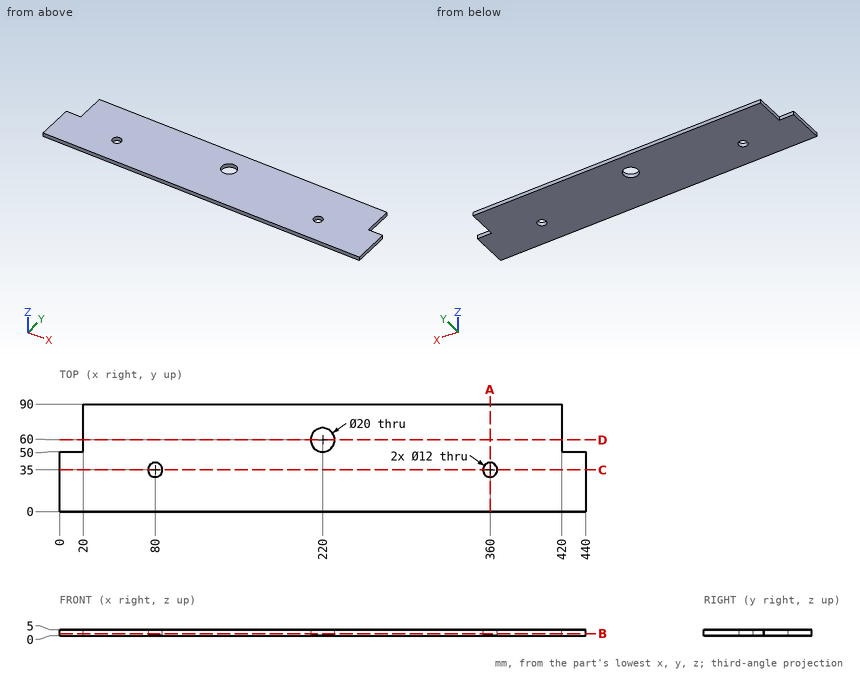
The figure shows three views and two pictorial views of one solid part (mm, origin at its lowest corner). Answer the questions. Give positions to 0.01 mm unless a question says otherwise; leave off trailing zeros. Write each loop counter-clockwise with the first axis right and the second up, starting at its lowest first coordinate (ties: lowest second). Pieces come first, ordered by that corner, then holes. Notation, with made-up numbers: (2.5, 59) -> (16.5, 59) arc R20 cw to (16.5, 75) -> close; hole circle Ø7 at (49, 7). An arc over 180 degrees is marked (long way). Answer as a JSON object with one key per item and string values.
1) Section A-A on x = 360 is taken. Write down the section's boundary in (y, z), then the cut area to 3 significant figures.
Findings below:
{"outline": "(0, 0) -> (29, 0) -> (29, 5) -> (0, 5) -> close; (41, 0) -> (90, 0) -> (90, 5) -> (41, 5) -> close", "area": "390 mm^2"}
2) Flat-ended cylindrical pins translate along their axes: pin 1 Ø16 at (x, y) = (220, 60) entering from -Z; pin 2 Ø2.5 at (x, z) = (429.5, 1.5) entering from +Y; pin 3 Ø3 at (y, z) = (74.5, 2) entering from -X. Find the tip coordinate at first contact, or state that the pin passes through.
Findings below:
{"pin 1": "passes through", "pin 2": "stops at y = 50", "pin 3": "stops at x = 20"}
3) Section B-B on z = 1.7 is taken. Write down the section's boundary in (x, y), then the cut area to 3 significant figures.
Findings below:
{"outline": "(0, 0) -> (440, 0) -> (440, 50) -> (420, 50) -> (420, 90) -> (20, 90) -> (20, 50) -> (0, 50) -> close; hole circle Ø12 at (80, 35); hole circle Ø20 at (220, 60); hole circle Ø12 at (360, 35)", "area": "37,500 mm^2"}
4) Section D-D on y = 60 is taken. Write down the section's boundary in (x, z), then the cut area to 3 significant figures.
Findings below:
{"outline": "(20, 0) -> (210, 0) -> (210, 5) -> (20, 5) -> close; (230, 0) -> (420, 0) -> (420, 5) -> (230, 5) -> close", "area": "1,900 mm^2"}
5) Section C-C on y = 35 is taken. Write down the section's boundary in (x, z).
Findings below:
{"outline": "(0, 0) -> (74, 0) -> (74, 5) -> (0, 5) -> close; (86, 0) -> (354, 0) -> (354, 5) -> (86, 5) -> close; (366, 0) -> (440, 0) -> (440, 5) -> (366, 5) -> close"}
6) Straight lines are drawn through the part: probe 1 along Y at (x, z) = (80, 2.7); probe 2 along Y at (x, z) = (220, 1.85); probe 3 along X at (y, z) = (39.5, 0.65). For each, find the intervals that lie inside material, in ascending order. Write a range as from..to.
Findings below:
{"probe 1": "y = 0..29, 41..90", "probe 2": "y = 0..50, 70..90", "probe 3": "x = 0..76.03, 83.97..356.03, 363.97..440"}
